Part print with two shaded views. Sizes in mm from the minimum x, y, z corner. Coordinates: 2 decimals unless noted, no trailing zeros. Loops run counter-clockwise (first coordinate to the right, second up) from the corner with the lowest first, then second, coordinate; pieces in that order, holes last. Notation, with made-up numbers: (-29, -33.5) -> (26, -33.5) arc R18 ccw to (26, -12.5) -> close; hole circle Ø8 at (9.5, -39.75). An arc over 180 degrees is marked (long way). Write each question's results on one line, items separated by ' | '.
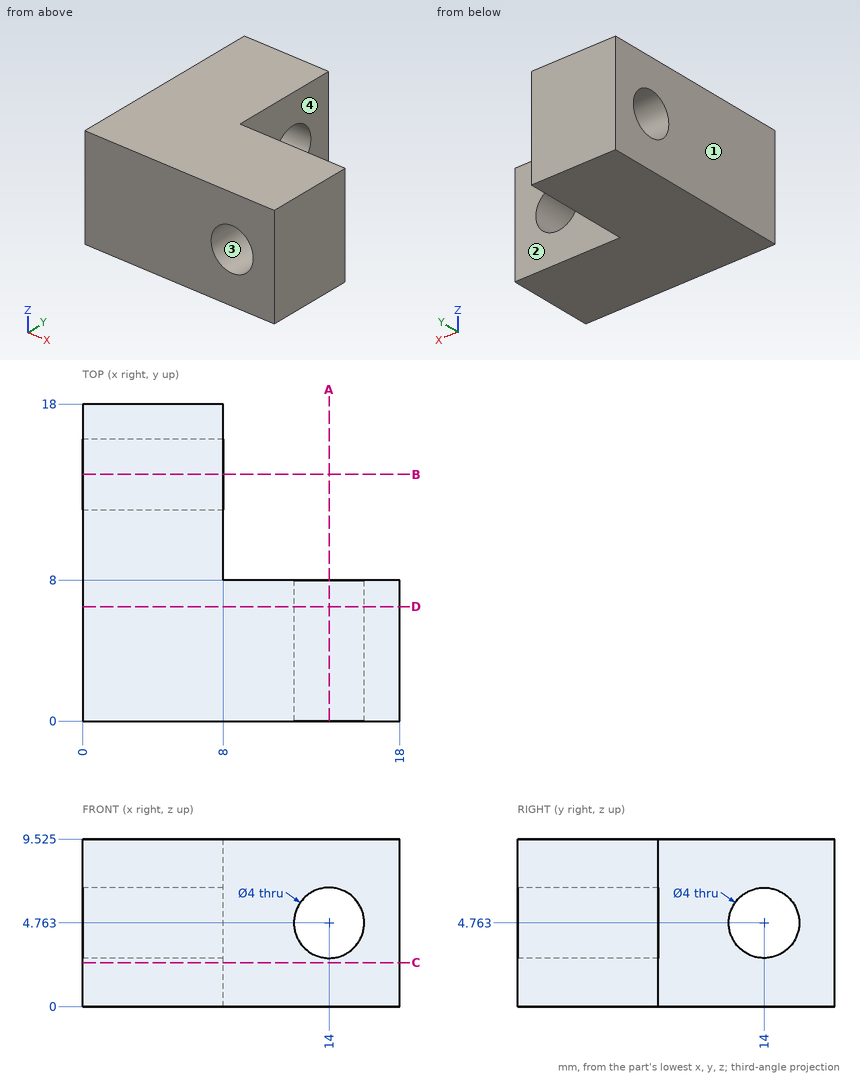
Q1. Cut at D-D on y = 6.5. Write the cut outline in (x, z) (1 decimal), and give its area (3 significant figures).
Results are:
outline: (0, 0) -> (18, 0) -> (18, 9.5) -> (0, 9.5) -> close; hole circle Ø4 at (14, 4.8) | area: 159 mm^2
Q2. Cut at A-A on x = 14. Write the cut outline in (y, z) (1 decimal), and give its area (3 significant figures).
Results are:
outline: (0, 0) -> (8, 0) -> (8, 2.8) -> (0, 2.8) -> close; (0, 6.8) -> (8, 6.8) -> (8, 9.5) -> (0, 9.5) -> close | area: 44.2 mm^2
Q3. Drop flat-ended pins along their axis: pin 1 (3 mm diameter, centred on x = 15.5, z = 6.5, fed in from +Y); pin 2 (1 mm diameter, centred on y = 11, z = 8, fed in from +X). Give the stop position or say it passes through.
Results are:
pin 1: y = 8 | pin 2: x = 8
Q4. Cut at C-C on z = 2.5. Write the cut outline in (x, y), and give its area (3 significant figures).
Results are:
outline: (0, 0) -> (18, 0) -> (18, 8) -> (8, 8) -> (8, 18) -> (0, 18) -> close | area: 224 mm^2
Q5. Pull direction X, two halves, no side cores. Call the marked faces 1, 2, 3 and 4: +X half, -X half, draft (parallel to the pull), parting line (faces both ways), or undercut.
Results are:
face 1: -X half | face 2: draft | face 3: undercut | face 4: +X half
Q6. Wall check: L1, parallel to Z at x = 3, y = 14 (1 decimal); L2, parallel to Y at x = 14, z = 1.25. Give the ranges that are in metal, low to high. Write a range as from..to.
Results are:
L1: 0..2.8, 6.8..9.5 | L2: 0..8
